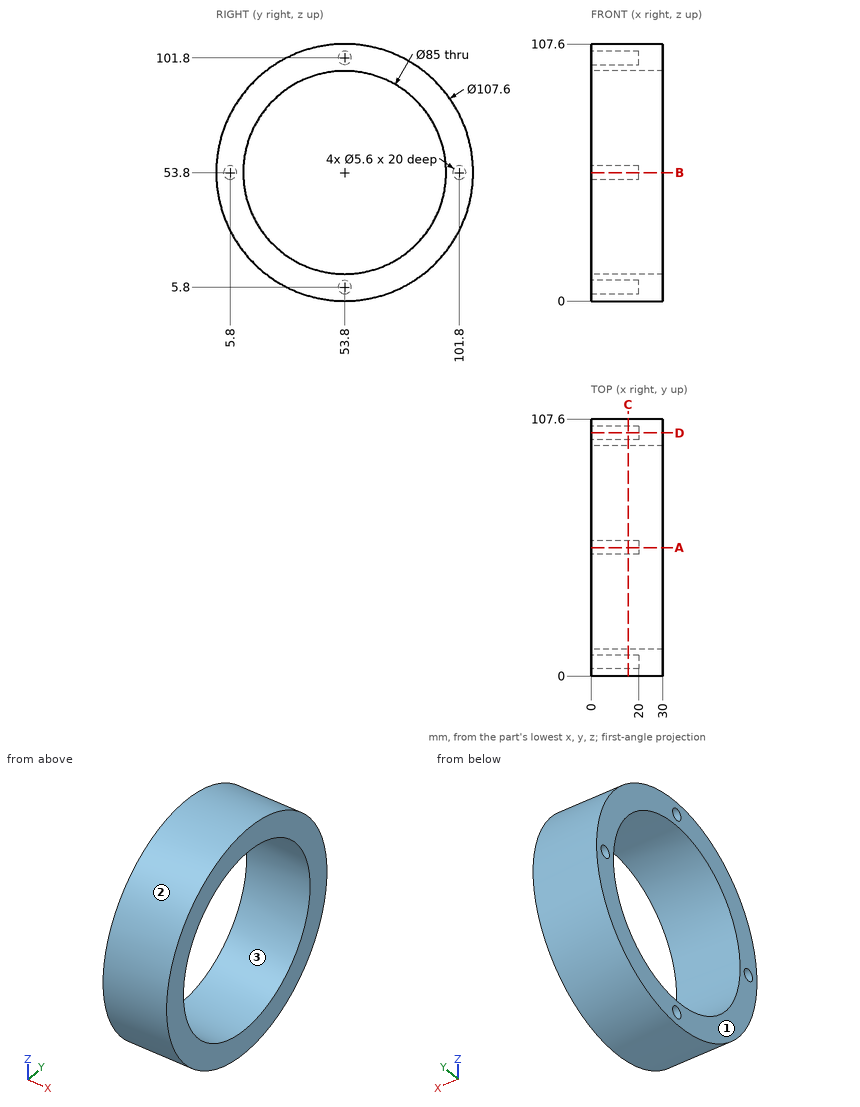
Job drawing, mm, ordinate dimensions from the low corner. One solid piece. Coordinates: 2 decimals unless noted, no trailing zeros. Loops run counter-clockwise (first coordinate to the right, second up) from the corner with the lowest first, then second, coordinate; pieces in that order, holes last. Notation, with made-up numbers: (43, 89) - (68, 89) arc R34 ccw to (68, 128) - close; hole circle Ø2 at (-21, 87). An arc over 180 degrees is marked (long way). Answer as a JSON object with one key per item and string values. Group by question number.
(1) Flat gauge pins, fed straight in: pin 1 (5 mm diameter, centred on x = 18, z = 15.5, fed in from +Y); pin 2 (6 mm diameter, centred on y = 54, z = 5, fed in from -X); pin 3 (3.5 mm diameter, centred on y = 101.8, z = 53.8, fed in from -X); pin 4 (6 mm diameter, centred on x = 8, z = 92, fed in from -Y). Where does each tip first touch, or does it go through?
(2) Cut at D-D (y = 101.8). Give the cut face in (x, z), then the cut area to 3 significant figures.
(3) Probe line 1 along Y through (x, z) = (15.5, 53.8); line 2 along Y through (x, z) = (21, 53.8); line 3 along Z through (x, y) = (7.5, 70.5). List the from-to ranges inside material, lowest first.
(4) Cut at A-A (y = 53.8). Give the cut face in (x, z).
(5) Two-plate mould, pull along Z, no slides. Class the marked faces 1, 2 and 3: released by +Z, released by -Z, zero draft, split by the parting line, or undercut.
(6) Cut at C-C (x = 15.5). Give the cut face in (y, z), then the cut area to 3 significant figures.
Geometry says:
{
 "1": {"pin 1": "stops at y = 93.96", "pin 2": "stops at x = 0", "pin 3": "stops at x = 20", "pin 4": "stops at y = 13.11"},
 "2": {"outline": "(0, 29.5) - (30, 29.5) - (30, 78.1) - (0, 78.1) - (0, 56.6) - (20, 56.6) - (20, 51) - (0, 51) - close", "area": "1,350 mm^2"},
 "3": {"line 1": "y = 0 to 3, 8.6 to 11.3, 96.3 to 99, 104.6 to 107.6", "line 2": "y = 0 to 11.3, 96.3 to 107.6", "line 3": "z = 2.66 to 14.72, 92.88 to 104.94"},
 "4": {"outline": "(0, 0) - (30, 0) - (30, 11.3) - (0, 11.3) - (0, 8.6) - (20, 8.6) - (20, 3) - (0, 3) - close; (0, 96.3) - (30, 96.3) - (30, 107.6) - (0, 107.6) - (0, 104.6) - (20, 104.6) - (20, 99) - (0, 99) - close"},
 "5": {"face 1": "zero draft", "face 2": "split by the parting line", "face 3": "undercut"},
 "6": {"outline": "circle Ø107.6 at (53.8, 53.8); hole circle Ø5.6 at (5.8, 53.8); hole circle Ø85 at (53.8, 53.8); hole circle Ø5.6 at (53.8, 5.8); hole circle Ø5.6 at (53.8, 101.8); hole circle Ø5.6 at (101.8, 53.8)", "area": "3,320 mm^2"}
}
